Could you check a few things on this drawing? It's one solid part, dimensions in mm from its lowest x, y, z. A direction names the side the tool comes from. Round coordinates to 2 decimals unless told otherwise and drop trailing zeros. Write each loop counter-clockwise with the first axis right and the second up, starting at its lowest first coordinate (ties: lowest second). Pieces come first, ordered by that corner, then holes. Notation, with made-up numbers: (-22, 71.25) - (14, 71.25) arc R18 cw to (14, 102.25) - close; hole circle Ø2 at (71, 35). An arc over 180 degrees is marked (long way). Write item = value, one per line. Start each with the question number.
Item 1: If we section it at B-B (x = 100): Please give me the cut outline in (y, z) (3 decimals).
Item 2: Thinking about a two-plate mould opening in Z: for the marked faces 1, 2, 3 and 4, which applies, pulls with the +Z half, pulls with the -Z half, needs draft (parallel to the pull), parting line crosses it, or undercut?
Item 3: If I drill on line 1 along Z through (x, y) = (90.5, 13) (3 decimals); line 2 along Y through (x, z) = (158, 2); line 3 along Y through (x, z) = (70.5, 31) (3 decimals), over which ranges is the centre line in solid material (lowest first)? Write a range as [from, to].
Item 4: If we section it at A-A (y = 33.5): Please give me the cut outline in (x, z) (3 decimals), and give its area (3 significant figures).
Item 5: If we section it at C-C (z = 19.05): Please give me the cut outline in (x, y) (3 decimals).
Item 6: If we section it at D-D (z = 26): Please give me the cut outline in (x, y) (3 decimals).
Item 7: Which directions (+Z, -Z, +X, -X, +Y, -Y) give clear straight access to the entire face, cutting with the end or side of a thin tool? Please do the marked faces 5 and 6.
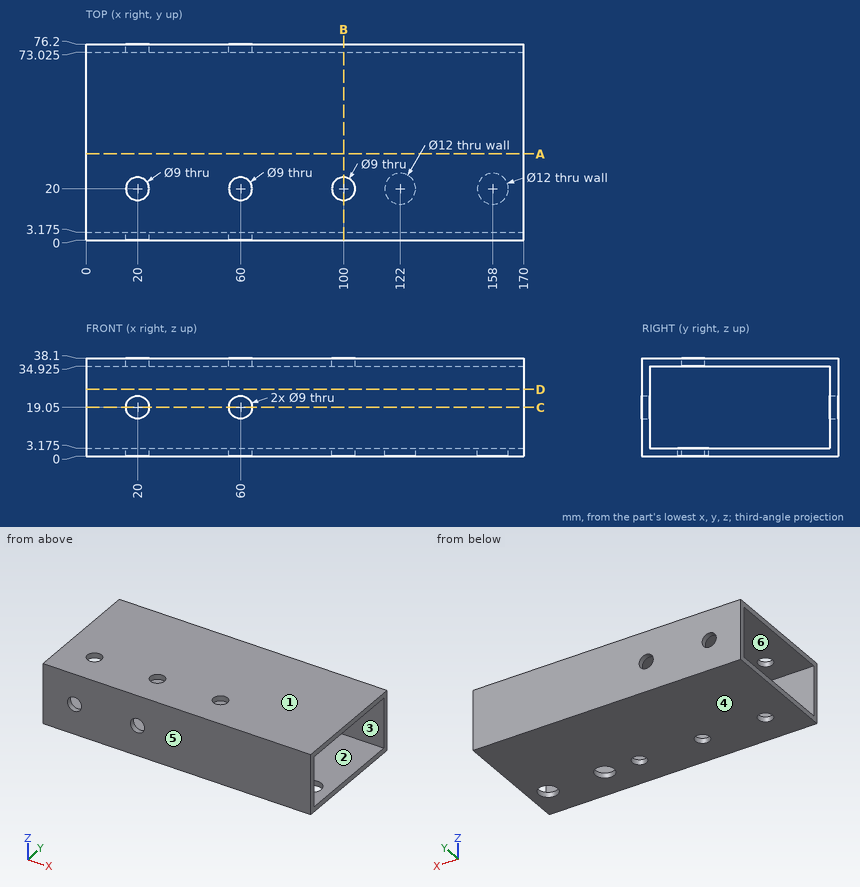
Reply:
q1.outline = (0, 0) - (15.5, 0) - (15.5, 3.175) - (3.175, 3.175) - (3.175, 34.925) - (15.5, 34.925) - (15.5, 38.1) - (0, 38.1) - close; (24.5, 0) - (76.2, 0) - (76.2, 38.1) - (24.5, 38.1) - (24.5, 34.925) - (73.025, 34.925) - (73.025, 3.175) - (24.5, 3.175) - close
q2.face_1 = pulls with the +Z half
q2.face_2 = undercut
q2.face_3 = undercut
q2.face_4 = pulls with the -Z half
q3.line_1 = [0, 3.175], [34.925, 38.1]
q3.line_2 = [0, 14], [26, 76.2]
q3.line_3 = [0, 3.175], [73.025, 76.2]
q4.outline = (0, 0) - (170, 0) - (170, 3.175) - (0, 3.175) - close; (0, 34.925) - (170, 34.925) - (170, 38.1) - (0, 38.1) - close
q4.area = 1,080 mm2
q5.outline = (0, 0) - (15.5, 0) - (15.5, 3.175) - (0, 3.175) - close; (0, 73.025) - (15.5, 73.025) - (15.5, 76.2) - (0, 76.2) - close; (24.5, 0) - (55.5, 0) - (55.5, 3.175) - (24.5, 3.175) - close; (24.5, 73.025) - (55.5, 73.025) - (55.5, 76.2) - (24.5, 76.2) - close; (64.5, 0) - (170, 0) - (170, 3.175) - (64.5, 3.175) - close; (64.5, 73.025) - (170, 73.025) - (170, 76.2) - (64.5, 76.2) - close
q6.outline = (0, 0) - (170, 0) - (170, 3.175) - (0, 3.175) - close; (0, 73.025) - (170, 73.025) - (170, 76.2) - (0, 76.2) - close
q7.face_5 = +Z, -Z, +X, -X, -Y
q7.face_6 = +X, -X
